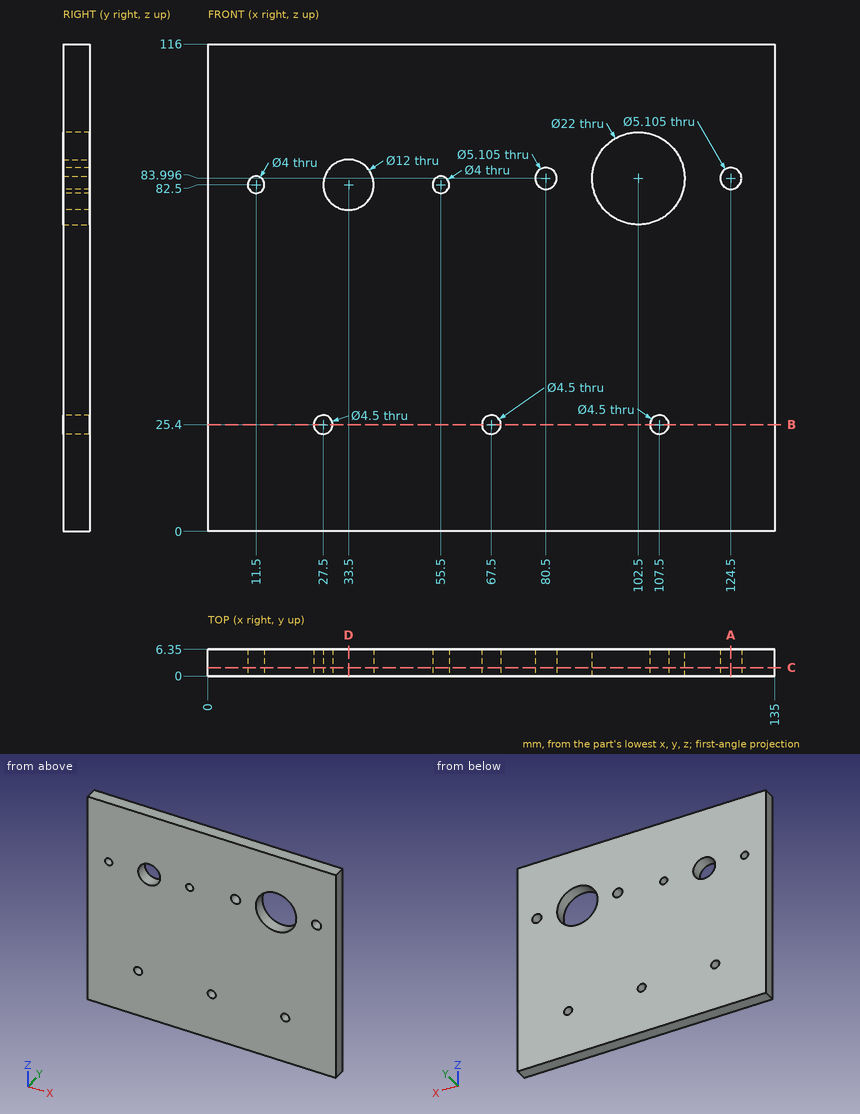
Verification items for this drawing (mm, ordinates from the low corner). Coordinates: 2 decimals unless noted, no trailing zeros. Loops run counter-clockwise (first coordinate to the right, second up) from the corner with the lowest first, then second, coordinate; pieces in that order, holes last. Notation, with made-up numbers: (10.5, -30.75) - (54.5, -30.75) arc R22 cw to (54.5, -16.75) - close; hole circle Ø11 at (-36, 76). An arc over 180 degrees is marked (long way). One line per item, written item: value. Start each with the question number.
(1) Material ranges on line 1 (X direction, y = 2.25, z = 25.4); line 2 (Z direction, x = 11.5, y = 2.5); line 3 (Z direction, x = 33.5, y = 3.75), recorded low to high. Write a range as [from, to].
(2) Cross-section at B-B on z = 25.4. Enter the section's corners in (x, y).
(3) Cross-section at C-C on y = 2. Count the separate pieces of the cut face and the enclosed holes in it, plus the area to 3 significant figures.
(4) Cross-section at A-A on x = 124.5. Enter the section's corners in (y, z), plus the area to 3 significant figures.
(5) Cross-section at D-D on x = 33.5. Enter the section's corners in (y, z).
(6) Depth check by flat-ended pin: P1, Ø4, axis at x = 67.5, z = 25.4, coming from the -Y side. Enter the tip coordinate at first touch or a pass-through.
Results below:
1. line 1: x = [0, 25.25], [29.75, 65.25], [69.75, 105.25], [109.75, 135]
1. line 2: z = [0, 80.5], [84.5, 116]
1. line 3: z = [0, 76.5], [88.5, 116]
2. outline: (0, 0) - (25.25, 0) - (25.25, 6.35) - (0, 6.35) - close; (29.75, 0) - (65.25, 0) - (65.25, 6.35) - (29.75, 6.35) - close; (69.75, 0) - (105.25, 0) - (105.25, 6.35) - (69.75, 6.35) - close; (109.75, 0) - (135, 0) - (135, 6.35) - (109.75, 6.35) - close
3. separate pieces: 1
3. enclosed holes: 9
3. area: 15,100 mm2
4. outline: (0, 0) - (6.35, 0) - (6.35, 81.44) - (0, 81.44) - close; (0, 86.55) - (6.35, 86.55) - (6.35, 116) - (0, 116) - close
4. area: 704 mm2
5. outline: (0, 0) - (6.35, 0) - (6.35, 76.5) - (0, 76.5) - close; (0, 88.5) - (6.35, 88.5) - (6.35, 116) - (0, 116) - close
6. P1: passes through
